Verification items for the finished model (mm, model axes). A direction names the side the tool comes from. Round coordinates to 2 decimals unless told otherwise and drop trailing zeros. Write each loop counter-clockwise with the first axis right and the second up, starting at its lowest first coordinate (ties: lowest second). Pieces come first, ordered by that corner, then holes. Notation, with made-up numbers: (49.25, 19) - (101.25, 19) arc R8 ccw to (101.25, 29) - close; hole circle Ø9 at (84.5, 35.5). An arc over 180 degrees is marked (long way). Answer as a JSON object with one key per item and string values.
```python
from build123d import *

# Parameters (mm, degrees)
SKETCH2_R           = 50
BOSS_EXTRUDE1_DEPTH = 17
SKETCH4_R           = 6.25
CUT_EXTRUDE1_DEPTH  = 17
SKETCH7_R           = 4
CUT_EXTRUDE2_DEPTH  = 5
SKETCH8_W           = 7.099474729
SKETCH8_H           = 14.03212915
CUT_EXTRUDE3_DEPTH  = 5
CUT_EXTRUDE4_DEPTH  = 3
CUT_EXTRUDE5_DEPTH  = 3


with BuildPart() as part:
    # Sketch2 → Boss-Extrude1 (new body)
    with BuildSketch(Plane(origin=(0, 0, 0), x_dir=(1, 0, 0), z_dir=(0, 1, 0))):
        with Locations(Location((0, 0, 0), (0, 0, 270))):
            Circle(SKETCH2_R)
    extrude(amount=BOSS_EXTRUDE1_DEPTH)

    # Sketch4 → Cut-Extrude1 (cut)
    with BuildSketch(Plane(origin=(0, 17, 0), x_dir=(1, 0, 0), z_dir=(0, 1, 0))):
        with Locations(Location((0, 0, 0), (0, 0, 270))):
            Circle(SKETCH4_R)
    extrude(amount=-CUT_EXTRUDE1_DEPTH, mode=Mode.SUBTRACT)

    # Sketch7 → Cut-Extrude2 (cut)
    with BuildSketch(Plane(origin=(0, 17, 0), x_dir=(1, 0, 0), z_dir=(0, 1, 0))):
        with Locations(Location((-10.75, -7.75, 0), (0, 0, 270))):
            Circle(SKETCH7_R)
    cut_extrude2 = extrude(amount=-CUT_EXTRUDE2_DEPTH, mode=Mode.SUBTRACT)

    # Mirror1: Cut-Extrude2 across plane
    add(cut_extrude2.mirror(Plane(origin=(0, 0, 0), x_dir=(0, 0, 1), z_dir=(1, 0, 0))), mode=Mode.SUBTRACT)

    # Sketch8 → Cut-Extrude3 (cut)
    with BuildSketch(Plane(origin=(0, 17, 0), x_dir=(1, 0, 0), z_dir=(0, 1, 0))):
        with Locations((0.370179164, -12.396855376)):
            Rectangle(SKETCH8_W, SKETCH8_H)
    extrude(amount=-CUT_EXTRUDE3_DEPTH, mode=Mode.SUBTRACT)

    # Sketch9 → Cut-Extrude4 (cut)
    with BuildSketch(Plane(origin=(0, 17, 0), x_dir=(1, 0, 0), z_dir=(0, 1, 0))):
        Polygon((-31.112706744, 17), (-8.372e-06, 48.112698372), (31.11269, 17), (-8.372e-06, -14.112698372), align=None)
    extrude(amount=-CUT_EXTRUDE4_DEPTH, mode=Mode.SUBTRACT)

    # Sketch6 → Cut-Extrude5 (cut)
    with BuildSketch(Plane(origin=(0, 17, 0), x_dir=(1, 0, 0), z_dir=(0, 1, 0))):
        Polygon((-5.977874391, 23.042765738), (5.977874391, 10.957234262), (25.17254203, 29.945776443), (13.216793249, 42.03130792), align=None)
    extrude(amount=-CUT_EXTRUDE5_DEPTH, mode=Mode.SUBTRACT)


solid = part.part
```
Q1. Section check B-B, the plane y = 6.25. Record the cut outline in (x, z), then the cut area to 3 significant figures.
Geometry check:
{"outline": "circle Ø100 at (0, 0); hole circle Ø12.5 at (0, 0)", "area": "7,730 mm2"}
Q2. Gauge pin test, flat ends, axial feed: P1, Ø8, axis at x = -1, z = 12.5, coming from the +Y side; P2, Ø6.5, axis at x = -10.75, z = 7.75, coming from the +Y side; P3, Ø3, axis at y = 13, z = -12.5, coming from the +X side (3 decimals); P4, Ø5.5, axis at y = 14, z = 16, coming from the +X side. Record the tip position at first contact, or that the pin passes through.
Geometry check:
{"P1": "stops at y = 17", "P2": "stops at y = 12", "P3": "stops at x = 48.775", "P4": "stops at x = 48.21"}
Q3. Section check C-C, the plane z = -21.5. Record the cut outline in (x, y).
Geometry check:
{"outline": "(-45.14, 0) - (45.14, 0) - (45.14, 17) - (26.61, 17) - (26.61, 14) - (-26.61, 14) - (-26.61, 17) - (-45.14, 17) - close"}
Q4. Section check A-A, the plane z = 0. Record the cut outline in (x, y), then the cut area to 3 significant figures.
Geometry check:
{"outline": "(-50, 0) - (-6.25, 0) - (-6.25, 14) - (-14.11, 14) - (-14.11, 17) - (-50, 17) - close; (6.25, 0) - (50, 0) - (50, 17) - (14.11, 17) - (14.11, 14) - (6.25, 14) - close", "area": "1,440 mm2"}
Q5. Material ranges on line 1 along Z through (x, y) = (10.75, 15.15); line 2 along X through (y, z) = (4.75, 0); line 3 along X through (y, z) = (13.3, 7.75), recorded low to high. Write a range as [from, to].
Geometry check:
{"line 1": "z = [-48.83, -39.59], [3.36, 3.75], [11.75, 48.83]", "line 2": "x = [-50, -6.25], [6.25, 50]", "line 3": "x = [-49.4, -14.75], [-6.75, -3.18], [3.92, 6.75], [14.75, 49.4]"}
Q6. Release check for a two-part mould opening along Z. For faces 3 (the cylindrical face through (15.02, 8.38, 47.69)), 4 (the flat face through (1, 17, 22)), 5 (the flat face through (11, 12, 8)) record: released by +Z, released by -Z, zero draft, split by the parting line, or undercut.
Geometry check:
{"face 3": "split by the parting line", "face 4": "zero draft", "face 5": "undercut"}
Q7. Section check D-D, the plane x = 38. Record the cut outline in (y, z).
Geometry check:
{"outline": "(0, -32.5) - (17, -32.5) - (17, 32.5) - (0, 32.5) - close"}
Q8. Set-up check for faces 1 (the flat face through (26.316, 15.521, -21.797)), 2 (the cylindrical face through (0.275, 7.098, -6.244)): record each of +Z, -Z, +X, -X, +Y, -Y from which the full face is reachable in a straight line by a thin tool's end or side.
Geometry check:
{"face 1": "+Y", "face 2": "+Y, -Y"}
